For this review, use the dimensioned drawing (mm, ordinates from the lowest corner) and the shaded views. A direction names the side the tool comes from. Round coordinates to 2 decimals unless told otherwise and drop trailing zeros. Loops run counter-clockwise (first coordinate to the right, second up) from the corner with the lowest first, then second, coordinate; pieces in that order, holes last. Notation, with made-up numbers: (40.5, 40.5) -> (89.5, 40.5) arc R29 cw to (89.5, 78.5) -> close; hole circle Ø8 at (47.5, -20.75). An arc over 180 degrees is marked (long way). Answer as CSV lines item,"result". Start each with the question number.
(1) Take a section at D-D, the plane x = 55.5. Write out the cut boundary in (y, z).
(2) Draft analysis for pull direction X (two halves, no side actions). For the marked faces 1, 2 and 3, state which applies: +X half, -X half, draft (parallel to the pull), parting line (faces both ways), or undercut.
(3) Take a section at A-A, the plane z = 26.5. Write out the cut boundary in (x, y), and give its area (3 significant figures).
(4) To check wall thickness, follow line 1 (Y direction, x = 163.9, z = 46.5); line 2 (X direction, y = 31.5, z = 35); line 3 (Z direction, x = 1.15, y = 32). State the ranges of each line that lie inside material, in increasing order. Write a range as from..to.
(5) Take a section at C-C, the plane y = 32. Write out the cut boundary in (x, z).
(6) Take a section at B-B, the plane x = 87.5. Write out the cut boundary in (y, z).
(7) Machinability: for the marked faces 4 and 5, which of the approach directions +Z, -Z, +X, -X, +Y, -Y give a long, thin tool a straight path to every point of the face, cutting with its end or side? Answer none if there is none.
(8) For P1, Ø13, axis at y = 21.5, z = 25, coming from the -X side; P2, Ø4, axis at x = 77.5, y = 22, coming from the +Z side, all flat-tipped, find the tip position at first contact; note any pin that passes through.
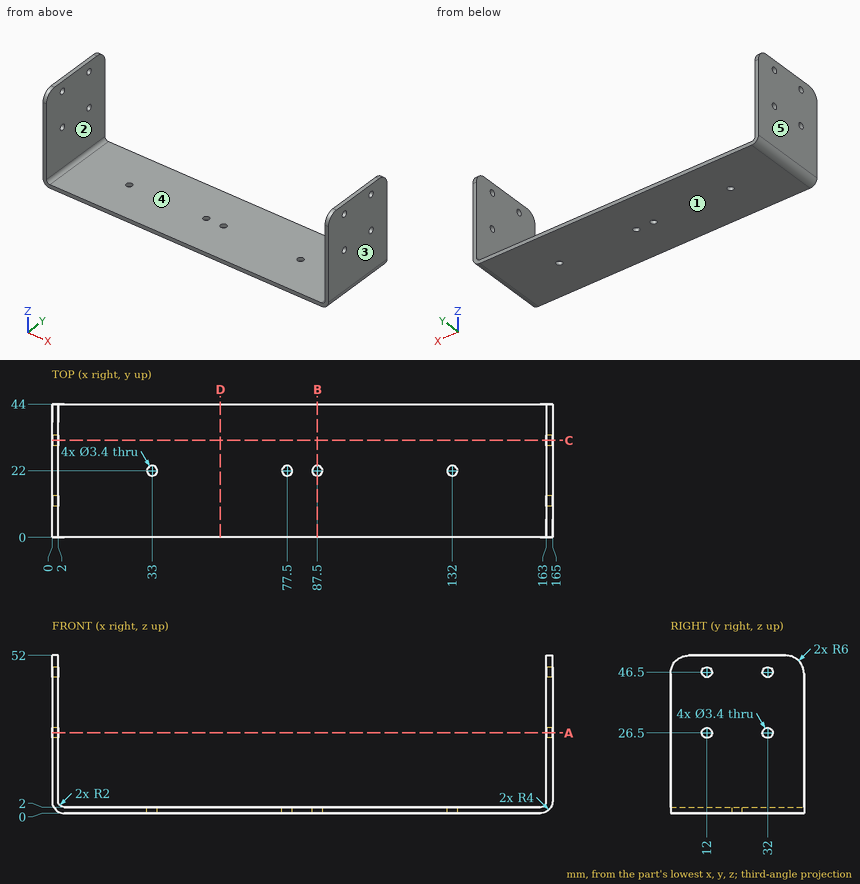
The answers:
1,outline,"(0, 0) -> (44, 0) -> (44, 2) -> (0, 2) -> close"
2,face 1,"draft"
2,face 2,"undercut"
2,face 3,"+X half"
3,outline,"(0, 0) -> (2, 0) -> (2, 10.3) -> (0, 10.3) -> close; (0, 13.7) -> (2, 13.7) -> (2, 30.3) -> (0, 30.3) -> close; (0, 33.7) -> (2, 33.7) -> (2, 44) -> (0, 44) -> close; (163, 0) -> (165, 0) -> (165, 10.3) -> (163, 10.3) -> close; (163, 13.7) -> (165, 13.7) -> (165, 30.3) -> (163, 30.3) -> close; (163, 33.7) -> (165, 33.7) -> (165, 44) -> (163, 44) -> close"
3,area,"149 mm²"
4,line 1,"0.02..10.3, 13.7..30.3, 33.7..43.98"
4,line 2,"0..2, 163..165"
4,line 3,"1.19..24.8, 28.2..44.8, 48.2..52"
5,outline,"(0, 4) arc R4 ccw to (4, 0) -> (161, 0) arc R4 ccw to (165, 4) -> (165, 24.8) -> (163, 24.8) -> (163, 4) arc R2 cw to (161, 2) -> (4, 2) arc R2 cw to (2, 4) -> (2, 24.8) -> (0, 24.8) -> close; (0, 28.2) -> (2, 28.2) -> (2, 44.8) -> (0, 44.8) -> close; (0, 48.2) -> (2, 48.2) -> (2, 52) -> (0, 52) -> close; (163, 28.2) -> (165, 28.2) -> (165, 44.8) -> (163, 44.8) -> close; (163, 48.2) -> (165, 48.2) -> (165, 52) -> (163, 52) -> close"
6,outline,"(0, 0) -> (20.3, 0) -> (20.3, 2) -> (0, 2) -> close; (23.7, 0) -> (44, 0) -> (44, 2) -> (23.7, 2) -> close"
7,face 4,"+Z, +Y, -Y"
7,face 5,"+Z, -Z, -X, +Y, -Y"
8,P1,"x = 0"
8,P2,"z = 2"
